Check sheet for the modelled part. Datum: model origin and axes. Units: mm. Give positions to 0.01 mm unless a question says otherwise; leave off trailing zeros. Loops run counter-clockwise (first coordinate to the right, second up) from the corner with the lowest first, then second, coordinate; pieces in that order, holes last. Notation, with made-up numbers: (14, -20) - (22, -20) arc R22 cw to (22, 15) - close; hole circle Ø10 at (84, 24.5). An arc over 180 degrees is marked (long way). Answer in a Markdown table with one row per item. Add a question column.
(1) Sectioned sample at C-C on x = 30. Enter the section's corners in (y, z), then the cut area to 3 significant figures.
(2) Thickness scan on L1, parallel to X at y = -0.5, z = 0; L2, parallel to X at y = -0.7, z = 10; L3, parallel to Z at x = 23, y = -0.05. Record the ranges inside material, lowest first.
(3) Sectioned sample at B-B on z = 10. Enter the section's corners in (x, y).
(4) Sectioned sample at D-D on y = -0.7. Enter the section's corners in (x, z), then the cut area to 3 significant figures.
(5) Sectioned sample at A-A on x = -14. Enter the section's corners in (y, z), then the cut area to 3 significant figures.
from build123d import *

# Parameters (mm, degrees)
ESQUISSE1_R               = 1.7
T_LE_DE_BASE_PLI_E1_DEPTH = 1


# Sheet-metal steps are written as plain solids
with BuildPart() as part:
    # Esquisse1 → Tôle de base pliée1 (new body)
    with BuildSketch(Plane(origin=(0, 0, 0), x_dir=(1, 0, 0), z_dir=(0, 1, 0))):
        with BuildLine():
            Line((-35, -15), (35, -15))
            Line((35, -15), (35, -5.5))
            Line((35, -5.5), (-11.602084238, -5.5))
            ThreePointArc((-11.602084238, -5.5), (-20, 0), (-11.602084238, 5.5))
            Line((-11.602084238, 5.5), (35, 5.5))
            Line((35, 5.5), (35, 15))
            Line((35, 15), (-35, 15))
            Line((-35, 15), (-35, -15))
        make_face()
        with Locations(Location((30, 10, 0), (0, 0, 270))):
            Circle(ESQUISSE1_R, mode=Mode.SUBTRACT)
        with Locations(Location((30, -10, 0), (0, 0, 90))):
            Circle(ESQUISSE1_R, mode=Mode.SUBTRACT)
        with Locations(Location((-30, 0, 0), (0, 0, 270))):
            Circle(ESQUISSE1_R, mode=Mode.SUBTRACT)
    extrude(amount=-T_LE_DE_BASE_PLI_E1_DEPTH)


solid = part.part
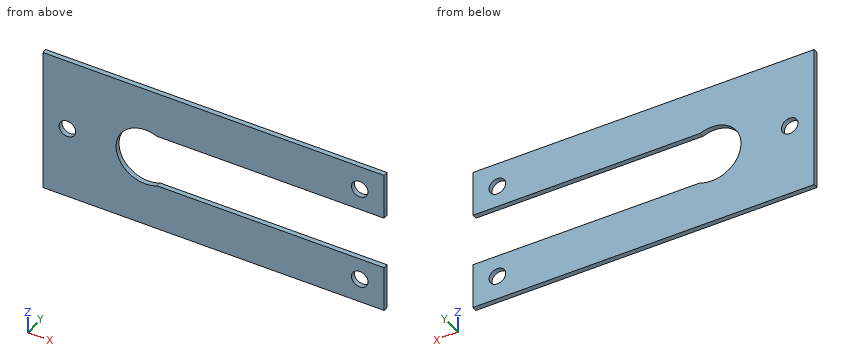
Reply:
| question | item | result |
|---|---|---|
| 1 | outline | (-1, -15) - (0, -15) - (0, -11.7) - (-1, -11.7) - close; (-1, -8.3) - (0, -8.3) - (0, -5.5) - (-1, -5.5) - close; (-1, 5.5) - (0, 5.5) - (0, 8.3) - (-1, 8.3) - close; (-1, 11.7) - (0, 11.7) - (0, 15) - (-1, 15) - close |
| 1 | area | 12.2 mm^2 |
| 2 | L1 | -35 to -31.7, -28.3 to -20 |
| 2 | L2 | -35 to 28.3, 31.7 to 35 |
| 2 | L3 | -15 to -5.5, 5.5 to 15 |
| 3 | outline | (-35, -1) - (28.3, -1) - (28.3, 0) - (-35, 0) - close; (31.7, -1) - (35, -1) - (35, 0) - (31.7, 0) - close |
| 4 | outline | (-35, -15) - (35, -15) - (35, -5.5) - (-11.6, -5.5) arc R6 cw (long way) to (-11.6, 5.5) - (35, 5.5) - (35, 15) - (-35, 15) - close; hole circle Ø3.4 at (-30, 0); hole circle Ø3.4 at (30, -10); hole circle Ø3.4 at (30, 10) |
| 4 | area | 1,480 mm^2 |
| 5 | outline | (-1, -15) - (0, -15) - (0, -6) - (-1, -6) - close; (-1, 6) - (0, 6) - (0, 15) - (-1, 15) - close |
| 5 | area | 18.0 mm^2 |
